Answer from the drawing. Dimensions are ordinates in mm from the lowest x, y and z of the part. A direction names the side the tool comes from. Coordinates: 2 decimals unless noted, no trailing zeros. Loops run counter-clockwise (first coordinate to the right, second up) from the corner with the lowest first, then second, coordinate; pieces in that order, holes last. Notation, with made-up numbers: (-5.5, 52) -> (46.5, 52) arc R21 cw to (46.5, 91) -> close; hole circle Ø7 at (-13.75, 18). An arc over 180 degrees is marked (long way). Answer as CSV lines item,"result".
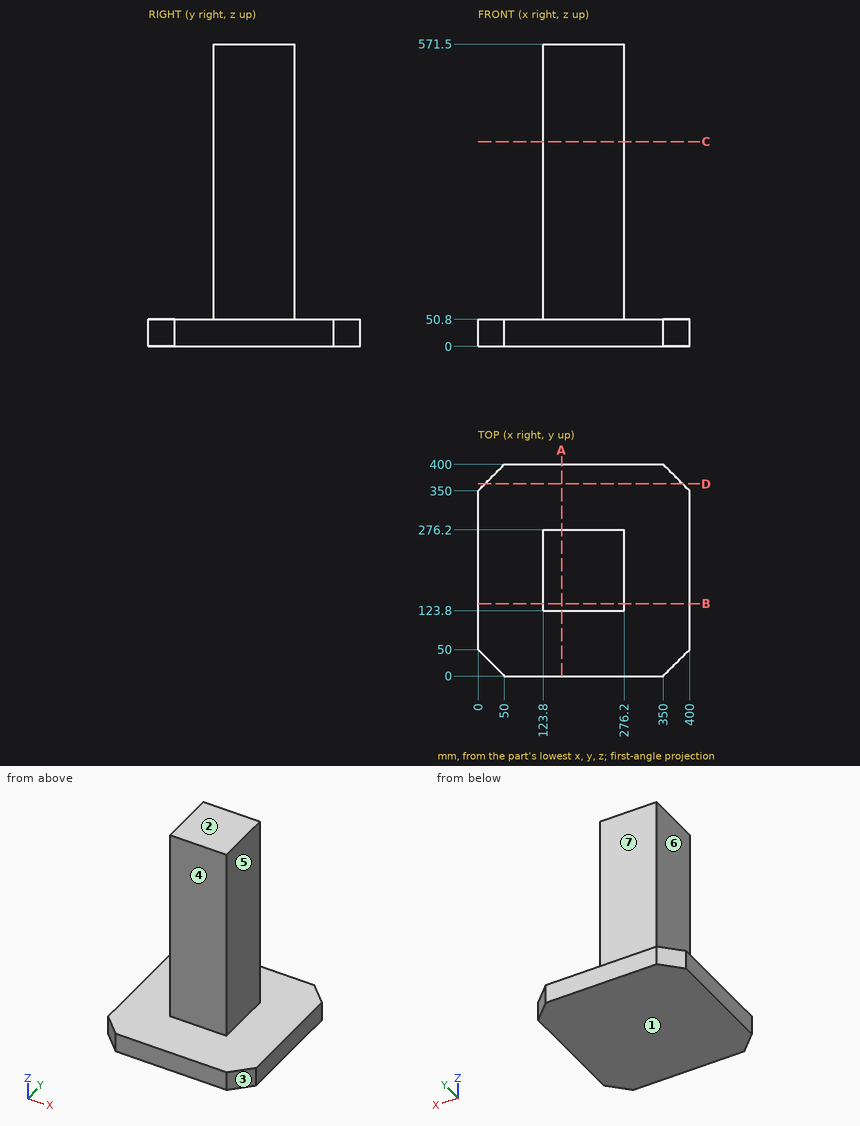
(1) Which of the six approach directions +Z, -Z, +X, -X, +Y, -Y give full straight-line access (tool end or side, diameter ignored) to the marked faces 4, 5, 6 and 7?
Computed values:
face 4,"+Z, +X, -X, -Y"
face 5,"+Z, +X, +Y, -Y"
face 6,"+Z, -X, +Y, -Y"
face 7,"+Z, +X, -X, +Y"
(2) Consider line 1 along Y through (x, z) = (166, 173); line 2 along Z through (x, y) = (252, 78.5). Determine where each line is inside the solid, lowest interval first.
Computed values:
line 1,"123.8 to 276.2"
line 2,"0 to 50.8"
(3) A cutting plane is placed at C-C, the plane z = 387. Write down the section's boundary in (x, y), and give its area (3 significant figures).
Computed values:
outline,"(123.8, 123.8) -> (276.2, 123.8) -> (276.2, 276.2) -> (123.8, 276.2) -> close"
area,"23,200 mm2"
(4) A cutting plane is placed at A-A, the plane x = 158. Write down the section's boundary in (y, z), and give its area (3 significant figures).
Computed values:
outline,"(0, 0) -> (400, 0) -> (400, 50.8) -> (276.2, 50.8) -> (276.2, 571.5) -> (123.8, 571.5) -> (123.8, 50.8) -> (0, 50.8) -> close"
area,"99,700 mm2"
(5) Flat-ended cylindrical pins translate along their axes: pin 1 Ø10 at (y, z) = (214.5, 184) entering from -X; pin 2 Ø3 at (y, z) = (213, 486) entering from +X; pin 3 Ø1.5 at (x, z) = (245, 70.5) entering from +Y. Find the tip coordinate at first contact, or state that the pin passes through.
Computed values:
pin 1,"x = 123.8"
pin 2,"x = 276.2"
pin 3,"y = 276.2"
(6) For a pull along Z with two mould halves and no side action, classify the marked faces 1, 2 and 3 as pulls with the +Z half, pulls with the -Z half, needs draft (parallel to the pull), parting line crosses it, or undercut.
Computed values:
face 1,"pulls with the -Z half"
face 2,"pulls with the +Z half"
face 3,"needs draft"
(7) A cutting plane is placed at D-D, the plane y = 363. Write down the section's boundary in (x, z).
Computed values:
outline,"(13, 0) -> (387, 0) -> (387, 50.8) -> (13, 50.8) -> close"
